```python
from build123d import *

# Parameters (mm, degrees)
BOSS_EXTRUDE1_DEPTH                                 = 22
SKETCH2_R                                           = 35
CUT_EXTRUDE1_DEPTH                                  = 18
SKETCH3_R                                           = 14
BOSS_EXTRUDE2_DEPTH                                 = 7
FILLET1_R                                           = 4
SKETCH4_R                                           = 10
CUT_EXTRUDE2_DEPTH                                  = 30
CHAMFER1_SIZE                                       = 2
M8X1_25_TAPPED_HOLE1_D                              = 6.8
M8X1_25_TAPPED_HOLE1_DEPTH                          = 29.75
M8X1_25_TAPPED_HOLE1_CSINK_D                        = 8.05
M8X1_25_TAPPED_HOLE1_CSINK_ANGLE                    = 90
M8X1_25_TAPPED_HOLE1_TIP                            = 2.042926105
CIRPATTERN1_COUNT                                   = 6
CSK_FOR_M8_COUNTERSUNK_FLAT_HEAD_SCREW1_D           = 6
CSK_FOR_M8_COUNTERSUNK_FLAT_HEAD_SCREW1_DEPTH       = 20
CSK_FOR_M8_COUNTERSUNK_FLAT_HEAD_SCREW1_CSINK_D     = 8
CSK_FOR_M8_COUNTERSUNK_FLAT_HEAD_SCREW1_CSINK_ANGLE = 90
CSK_FOR_M8_COUNTERSUNK_FLAT_HEAD_SCREW1_TIP         = 1.802581857


with BuildPart() as part:
    # Sketch1 → Boss-Extrude1 (new body)
    with BuildSketch(Plane.XY):
        with BuildLine():
            Line((-50, -59.5), (50, -59.5))
            Line((50, -59.5), (50, -49.5))
            Line((50, -49.5), (34, -49.5))
            ThreePointArc((34, -49.5), (31.171572875, -48.328427125), (30, -45.5))
            Line((30, -45.5), (30, -41.306779105))
            ThreePointArc((30, -41.306779105), (30.792252789, -37.405831617), (33.043478261, -34.122991434))
            ThreePointArc((33.043478261, -34.122991434), (47.217043986, -5.176944775), (39.652173913, 26.152535326))
            ThreePointArc((39.652173913, 26.152535326), (38.421945373, 28.784159388), (38, 31.658332237))
            Line((38, 31.658332237), (38, 47.5))
            Line((38, 47.5), (0, 47.5))
            ThreePointArc((0, 47.5), (-44.028922841, 17.824251834), (-33.043478261, -34.122991434))
            ThreePointArc((-33.043478261, -34.122991434), (-30.792252789, -37.405831617), (-30, -41.306779105))
            Line((-30, -41.306779105), (-30, -45.5))
            ThreePointArc((-30, -45.5), (-31.171572875, -48.328427125), (-34, -49.5))
            Line((-34, -49.5), (-50, -49.5))
            Line((-50, -49.5), (-50, -59.5))
        make_face()
    extrude(amount=BOSS_EXTRUDE1_DEPTH)

    # Sketch2 → Cut-Extrude1 (cut)
    with BuildSketch(Plane.XY.offset(22)):
        Circle(SKETCH2_R)
    extrude(amount=-CUT_EXTRUDE1_DEPTH, mode=Mode.SUBTRACT)

    # Sketch3 → Boss-Extrude2 (add)
    with BuildSketch(Plane(origin=(0, 0, 0), x_dir=(-1, 0, 0), z_dir=(0, 0, -1))):
        Circle(SKETCH3_R)
    extrude(amount=BOSS_EXTRUDE2_DEPTH)

    # Fillet1
    fillet1_edges = [part.edges().sort_by_distance(p)[0] for p in [
        (14, 0, 0),
    ]]
    fillet(fillet1_edges, radius=FILLET1_R)

    # Sketch4 → Cut-Extrude2 (cut, through all)
    with BuildSketch(Plane(origin=(0, 0, -7), x_dir=(-1, 0, 0), z_dir=(0, 0, -1))):
        Circle(SKETCH4_R)
    extrude(amount=-CUT_EXTRUDE2_DEPTH, mode=Mode.SUBTRACT)

    # Chamfer1
    chamfer1_edges = [part.edges().sort_by_distance(p)[0] for p in [
        (50, -54.5, 0),
        (-50, -54.5, 0),
        (-50, -54.5, 22),
        (50, -54.5, 22),
    ]]
    chamfer(chamfer1_edges, length=CHAMFER1_SIZE)

    # M8x1.25 Tapped Hole1
    with Locations(Plane(origin=(0, 47.5, 0), x_dir=(1, 0, 0), z_dir=(0, 1, 0))):
        with Locations((30.22415, -11)):
            CounterSinkHole(M8X1_25_TAPPED_HOLE1_D / 2, M8X1_25_TAPPED_HOLE1_CSINK_D / 2, depth=M8X1_25_TAPPED_HOLE1_DEPTH, counter_sink_angle=M8X1_25_TAPPED_HOLE1_CSINK_ANGLE)
            with Locations((0, 0, -(M8X1_25_TAPPED_HOLE1_DEPTH + M8X1_25_TAPPED_HOLE1_TIP / 2))):  # 118° drill point
                Cone(0, M8X1_25_TAPPED_HOLE1_D / 2, M8X1_25_TAPPED_HOLE1_TIP, mode=Mode.SUBTRACT)

    # Sketch10 → M6x1.0 Tapped Hole1 (revolve, cut)
    with BuildSketch(Plane(origin=(0, 40, 22), x_dir=(0, -1, 0), z_dir=(1, 0, 0))):
        Polygon((0, 0), (0, 16.502151548), (2.5, 15), (2.5, 0.525), (3.025, 0), align=None)
    m6x1_0_tapped_hole1 = revolve(axis=Axis((0, 40, 28.35), (0, 0, -1)), mode=Mode.SUBTRACT)

    # CirPattern1: M6x1.0 Tapped Hole1 ×6 about axis
    cirpattern1_axis = Axis((0, 0, 0), (0, 0, 1))
    for i in range(1, CIRPATTERN1_COUNT):
        add(m6x1_0_tapped_hole1.rotate(cirpattern1_axis, i * 360 / CIRPATTERN1_COUNT), mode=Mode.SUBTRACT)

    # CSK for M8 Countersunk Flat Head Screw1
    with Locations(Plane(origin=(0, -59.5, 0), x_dir=(-1, 0, 0), z_dir=(0, -1, 0))):
        with Locations((42, -11), (-42, -11)):
            CounterSinkHole(CSK_FOR_M8_COUNTERSUNK_FLAT_HEAD_SCREW1_D / 2, CSK_FOR_M8_COUNTERSUNK_FLAT_HEAD_SCREW1_CSINK_D / 2, depth=CSK_FOR_M8_COUNTERSUNK_FLAT_HEAD_SCREW1_DEPTH, counter_sink_angle=CSK_FOR_M8_COUNTERSUNK_FLAT_HEAD_SCREW1_CSINK_ANGLE)
            with Locations((0, 0, -(CSK_FOR_M8_COUNTERSUNK_FLAT_HEAD_SCREW1_DEPTH + CSK_FOR_M8_COUNTERSUNK_FLAT_HEAD_SCREW1_TIP / 2))):  # 118° drill point
                Cone(0, CSK_FOR_M8_COUNTERSUNK_FLAT_HEAD_SCREW1_D / 2, CSK_FOR_M8_COUNTERSUNK_FLAT_HEAD_SCREW1_TIP, mode=Mode.SUBTRACT)


solid = part.part
```
Could you check a few things on this model? Use its own coordinates, in mm. A direction names the side the tool comes from. Round coordinates to 2 decimals unless told otherwise and drop trailing zeros. Write each loop counter-clockwise with the first axis right and the second up, starting at its lowest first coordinate (ties: lowest second). Pieces come first, ordered by that corner, then holes.
(1) If I drill on probe 1 along X at (y, z) = (-52, 11); probe 2 along X at (y, z) = (20, 18); probe 3 along Z at (x, y) = (42, -53), over which ranges is the centre line in solid material (lowest first)?
Findings below:
probe 1: x = -50 to -45, -39 to 39, 45 to 50
probe 2: x = -43.08 to -37.14, -32.14 to -28.72, 28.72 to 32.14, 37.14 to 43.08
probe 3: z = 0 to 8, 14 to 22
(2) Suppose I cut it at B-B on x = -42. Write out the boundary of the cut face in (y, z).
Findings below:
outline: (-59.5, 0) - (-49.5, 0) - (-49.5, 8) - (-58.5, 8) - (-59.5, 7) - close; (-59.5, 15) - (-58.5, 14) - (-49.5, 14) - (-49.5, 22) - (-59.5, 22) - close; (-22.19, 0) - (22.19, 0) - (22.19, 22) - (-22.19, 22) - close
(3) Suppose I cut it at C-C on z = -2.5. Write out the boundary of the cut face in (x, y).
Findings below:
outline: circle Ø28.58 at (0, 0); hole circle Ø20 at (0, 0)
(4) Which directions (+Z, -Z, +X, -X, +Y, -Y) give clear straight access to the entire face, cutting with the end or side of a thin tool? Please do faces 5 (the face through (21, -29, 22)), 6 (the face through (0.96, 37.69, 14.34)), 7 (the face through (-12.932, -5.362, -5.479)).
Findings below:
face 5: +Z, +X, -X, +Y, -Y
face 6: +Z
face 7: -Z
(5) For pin 1 (12 mm diameter, centred on x = 0, y = 0, fed in from +Z); pin 2 (4 mm diameter, centred on y = -23, z = 17, fed in from +X); pin 3 (5 mm diameter, centred on y = 39.5, z = 8, fed in from +X); pin 4 (6 mm diameter, centred on y = 27.5, z = 12, fed in from -X), each with a flat end and sliding along its axis, tell me the tip position at first contact or that it passes through.
Findings below:
pin 1: passes through
pin 2: stops at x = 42.61
pin 3: stops at x = 38
pin 4: stops at x = -40.69
(6) Suppose I cut it at A-A on y = 0. Write out the boundary of the cut face in (x, z), and give its area (3 significant figures).
Findings below:
outline: (-47.5, 0) - (-18, 0) arc R4 cw to (-14, -4) - (-14, -7) - (-10, -7) - (-10, 4) - (-35, 4) - (-35, 22) - (-47.5, 22) - close; (10, -7) - (14, -7) - (14, -4) arc R4 cw to (18, 0) - (47.5, 0) - (47.5, 22) - (35, 22) - (35, 4) - (10, 4) - close
area: 813 mm2
(7) Thinking about a two-plate mould opening in X: for faces 1 (the face through (19, 47.5, 11)), 2 (the face through (-30, -43, 11)), 3 (the face through (34.21, -19.94, 5.76)), 4 (the face through (-36.75, -21.34, 14.34)), which applies, +X half, -X half, draft (parallel to the pull), parting line (faces both ways), or undercut?
Findings below:
face 1: draft
face 2: -X half
face 3: undercut
face 4: undercut
